Autodesk Inventor part; units mm, degrees
ref_plane "YZ Plane" through (0, 0, 0) normal (1, 0, 0) x (0, 1, 0)
ref_plane "XZ Plane" through (0, 0, 0) normal (0, 1, 0) x (-1, 0, 0)
ref_plane "XY Plane" through (0, 0, 0) normal (0, 0, 1) x (1, 0, 0)
sketch "スケッチ1" plane through (0, 0, 0) normal (1, 0, 0) x (0, 1, 0)
  line L0 (0.6302, 30) -> (-49.0748, 30)
  line L1 (0.6302, 0) -> (-66.7648, 0)
  line L2 (-49.0748, 30) -> (-66.7648, 0)
  line L3 (0.6302, 30) -> (0.6302, 0)
  line L4 (0.6302, 0) -> (0.6302, 30)
  point P0 (0, 0)
  dimension "d0" = 30
  dimension "d30" = 67.395
  dimension "d31" = 49.705
extrude "押し出し1" add sketch "スケッチ1" along normal blind 70
sketch "スケッチ7" plane through (0, -66.7648, 0) normal (0, 0, -1) x (-1, 0, 0)
  line L0 (0, 67.395) -> (-70, 67.395)
  line L1 (0, 0) -> (-70, 0)
  line L2 (-35, 67.395) -> (-35, 0)
  line L3 (-35, 0) -> (-35, 50)
  line L4 (-50, 50) -> (-20, 50)
  line L5 (-20, 50) -> (-20, 0)
  line L6 (-20, 0) -> (-50, 0)
  line L7 (-50, 0) -> (-50, 50)
  line L8 (-50, 50) -> (-20, 0) construction
  line L9 (-20, 50) -> (-50, 0) construction
  point P0 (0, 66.7648)
  point P1 (-35, 25)
  dimension "d32" = 50
  dimension "d33" = 30
extrude "押し出し4" cut sketch "スケッチ7" against normal blind 50
sketch "スケッチ8" plane through (0, 0.6302, 30) normal (0, 1, 0) x (1, 0, 0)
  line L0 (0, 30) -> (0, 0)
  line L1 (0, 0) -> (70, 0)
  line L2 (70, 30) -> (70, 0)
  line L3 (0, 30) -> (70, 30)
  line L4 (-15, 30) -> (85, 30)
  line L5 (85, 30) -> (85, -20)
  line L6 (85, -20) -> (-15, -20)
  line L7 (-15, -20) -> (-15, 30)
  line L8 (-15, 30) -> (85, -20) construction
  line L9 (85, 30) -> (-15, -20) construction
  point P0 (35, 5)
  dimension "d36" = 100
  dimension "d37" = 50
  dimension "d44" = 30
extrude "押し出し5" add sketch "スケッチ8" against normal blind 5 contours L0 L1 L2 L4 L5 L6 L7
sketch "スケッチ9" plane through (-15, 0.6302, 0) normal (0, 1, 0) x (1, 0, 0)
  line L0 (100, -50) -> (0, -50)
  line L1 (0, 0) -> (5, 0)
  line L2 (5, 0) -> (5, -50)
  line L3 (5, -50) -> (0, -50)
  line L4 (0, -50) -> (0, 0)
  line L5 (100, 0) -> (95, 0)
  line L6 (95, 0) -> (95, -50)
  line L7 (95, -50) -> (100, -50)
  line L8 (100, -50) -> (100, 0)
  point P0 (15, 0)
  dimension "d40" = 5
  dimension "d41" = 5
extrude "押し出し6" add sketch "スケッチ9" along normal blind 15
sketch "スケッチ10" plane through (-15, -4.3698, 50) normal (0, 0, 1) x (1, 0, 0)
  line L0 (95, 5) -> (5, 5)
  line L1 (5, 5) -> (5, 20)
  line L2 (0, 20) -> (5, 20)
  line L3 (0, 20) -> (0, 0)
  line L4 (100, 0) -> (0, 0)
  line L5 (100, 20) -> (100, 0)
  line L6 (95, 20) -> (100, 20)
  line L7 (95, 5) -> (95, 20)
  point P0 (15, 4.3698)
extrude "押し出し7" add sketch "スケッチ10" along normal blind 5
properties part number "知能ロボコン発射台支え" material "ABS プラスチック"
For this review, take the finished solid that the model builds, in its own axes (mm). A direction names the side the tool comes from. Round coordinates to 2 decimals unless told otherwise and drop trailing zeros. Order: outer loops, then holes, each group sorted by start corner. A loop starts at its lowest first (then second) coordinate and runs counter-clockwise, first axis right, second up.
Q1. Mouldability with a two-part tool opening along X and no side actions: class faces 4 (the flat face through (-10, 8, 27)), 5 (the flat face through (-15, 6, 27)), 6 (the flat face through (70, -29, 15)), 7 (the flat face through (82, 15.63, 27)) as pulls with the +X half, pulls with the -X half, needs draft (parallel to the pull), parting line crosses it, or undercut.
Findings below:
face 4: undercut
face 5: pulls with the -X half
face 6: pulls with the +X half
face 7: needs draft
Q2. We need section A-A, the plane y = -25.5. Give the boundary of the cut face in (x, z), plus the area to 3 significant figures.
Findings below:
outline: (0, 0) - (20, 0) - (20, 30) - (0, 30) - close; (50, 0) - (70, 0) - (70, 30) - (50, 30) - close
area: 1,200 mm2
Q3. We need section B-B, the plane y = 9.5. Give the boundary of the cut face in (x, z), plus the area to 3 significant figures.
Findings below:
outline: (-15, 0) - (-10, 0) - (-10, 55) - (-15, 55) - close; (80, 0) - (85, 0) - (85, 55) - (80, 55) - close
area: 550 mm2
Q4. Machinability: for faces 1 (the flat face through (0, -29, 15)), 2 (the flat face through (50, -37, 15)), 3 (the flat face through (36, 0.63, 27)), which of the approach directions +Z, -Z, +X, -X, +Y, -Y give a long, thin tool a straight path to every point of the face, cutting with its end or side? Answer none if there is none.
Findings below:
face 1: +Z, -Z, -X, -Y
face 2: +Z, -Z, -Y
face 3: +Z, -Z, +Y
Q5. We need section C-C, the plane x = 36. Give the boundary of the cut face in (y, z), plus the area to 3 significant figures.
Findings below:
outline: (-16.76, 0) - (0.63, 0) - (0.63, 55) - (-4.37, 55) - (-4.37, 30) - (-16.76, 30) - close
area: 647 mm2
Q6. Insertion check: P1, Ø9, axis at y = -20.5, z = 18, coming from the +X side; P2, Ø9, axis at y = -46.5, z = 19.5, coming from the -X side; P3, Ø4, axis at x = 37, y = -13.5, coming from the +Z side. Each pin has a flat end and moves straight along its axis. Give the tip position at first contact, or say it passes through.
Findings below:
P1: stops at x = 70
P2: stops at x = 0
P3: stops at z = 30
Q7. Wall thickness on line 1 (X direction, y = -48.5, z = 27.5); line 2 (X direction, y = 8.5, z = 42); line 3 (Y direction, x = 42, z = 35): over which ranges is each line inside the solid? List them lowest first.
Findings below:
line 1: x = 0 to 20, 50 to 70
line 2: x = -15 to -10, 80 to 85
line 3: y = -4.37 to 0.63
Q8. We need section D-D, the plane z = 34. Give the boundary of the cut face in (x, y), plus the area to 3 significant figures.
Findings below:
outline: (-15, -4.37) - (85, -4.37) - (85, 15.63) - (80, 15.63) - (80, 0.63) - (-10, 0.63) - (-10, 15.63) - (-15, 15.63) - close
area: 650 mm2
